Input: dimensioned drawing with shaded views. Units: mm. Origin: part minimum x, y, z. Round coordinates to 2 decimals unless told otherwise and drop trailing zeros. Loops run counter-clockwise (first coordinate to the right, second up) from the corner with the lowest first, then second, coordinate; pieces in that order, holes last. Notation, with made-up numbers: (62, 37) - (89, 37) arc R30 cw to (89, 73) - close; hole circle Ø5 at (20, 37). An arc over 180 degrees is marked (long way). Answer as CSV lines item,"result".
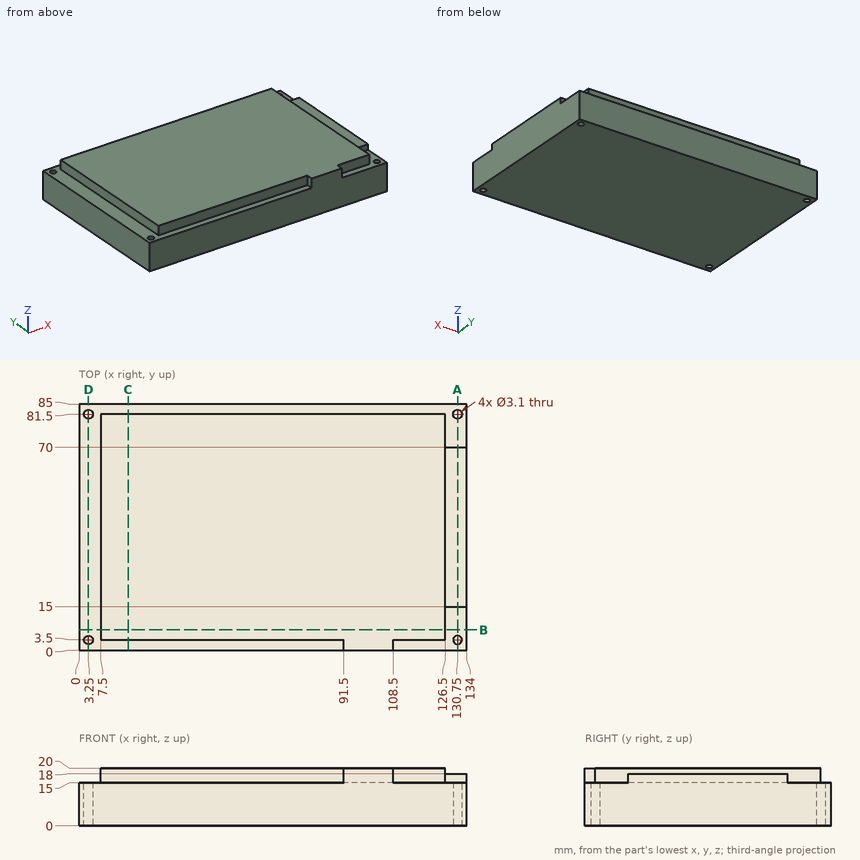
(1) Material intervals for line 1 along Y through (x, z) = (3.25, 11); line 2 along X through (y, z) = (81.5, 11.25); line 3 along Y through (x, z) = (40, 15.25), sorted ascending.
Findings below:
line 1,"0 to 1.95, 5.05 to 79.95, 83.05 to 85"
line 2,"0 to 1.7, 4.8 to 129.2, 132.3 to 134"
line 3,"3.5 to 81.5"
(2) Section C-C (x = 17). Output: boundary loops of the cut face in (y, z).
Findings below:
outline,"(0, 0) - (85, 0) - (85, 15) - (81.5, 15) - (81.5, 20) - (3.5, 20) - (3.5, 15) - (0, 15) - close"
(3) Section B-B (y = 7). Output: boundary loops of the cut face in (x, z).
Findings below:
outline,"(0, 0) - (134, 0) - (134, 15) - (126.5, 15) - (126.5, 20) - (7.5, 20) - (7.5, 15) - (0, 15) - close"
(4) Section D-D (x = 3.25). Output: boundary loops of the cut face in (y, z), and give its area (3 significant figures).
Findings below:
outline,"(0, 0) - (1.95, 0) - (1.95, 15) - (0, 15) - close; (5.05, 0) - (79.95, 0) - (79.95, 15) - (5.05, 15) - close; (83.05, 0) - (85, 0) - (85, 15) - (83.05, 15) - close"
area,"1,180 mm2"
(5) Pin query (flat end, axial travel): P1, Ø2.5, axis at x = 119, z = 18, coming from the -Y side; P2, Ø1.5, axis at x = 129, z = 17, coming from the +Y side; P3, Ø5, axis at x = 3.25, y = 81.5, coming from the +Z side. Return the tip coordinate at first contact, or that it passes through.
Findings below:
P1,"y = 3.5"
P2,"y = 70"
P3,"z = 15"
(6) Section A-A (x = 130.75). Output: boundary loops of the cut face in (y, z).
Findings below:
outline,"(0, 0) - (1.95, 0) - (1.95, 15) - (0, 15) - close; (5.05, 0) - (79.95, 0) - (79.95, 15) - (70, 15) - (70, 18) - (15, 18) - (15, 15) - (5.05, 15) - close; (83.05, 0) - (85, 0) - (85, 15) - (83.05, 15) - close"
